Could you check a few things on this model? Use its own coordinates, in mm. A direction names the side the tool comes from. Give positions to 0.01 mm unless a question says otherwise; leave off trailing zeros. Loops run counter-clockwise (first coordinate to the right, second up) from the corner with the lowest first, then second, coordinate; pieces in that order, holes last. Notation, with made-up numbers: M 6,54.25 L 38,54.25 A23 ccw 38,93.25 Z; hole C -32,79.5 d8. An arc over 180 degrees is marked long. Use CSV: the item, a comma, the result in double quotes.
```python
from build123d import *

# Parameters (mm, degrees)
F1_DEPTH    = 30
F2_T1_DEPTH = 40
F3_T1_DEPTH = 40
F4_T1_DEPTH = 40


# Not quite as in the source:
# - a fillet or chamfer that OpenCascade refuses, or shapes differently, is made with other operations: its cross-section is extruded or revolved along the edge and cut away or added


with BuildPart() as f1:
    # F0 (on Top) → F1 (new body)
    with BuildSketch(Plane.XY):
        Polygon((-20, 3), (-23, 3), (-23, -12), (-20, -12), (-20, 0), (0, 0), (0, -12), (0, -24.0508113056), (3, -24.0508113056), (3, -12), (3, 0), (19, 0), (22, 0), (22, 22.2248057965), (19, 22.2248057965), (19, 3), (3, 3), (3, 22.2248057965), (0, 22.2248057965), (0, 3), align=None)
    extrude(amount=F1_DEPTH)

    # F2: fillet of radius 2 on 2 edges, made by hand

    # F2_s2 → F2_t1 (cut)
    with BuildSketch(Plane.XY.offset(-5)):
        with BuildLine():
            ThreePointArc((2, -24.0508113056), (0.5857864376, -23.465024868), (0, -22.0508113056))
            Line((0, -22.0508113056), (0, -24.0508113056))
            Line((0, -24.0508113056), (2, -24.0508113056))
        make_face()
        with BuildLine():
            ThreePointArc((3, -22.0508113056), (2.4142135624, -23.465024868), (1, -24.0508113056))
            Line((1, -24.0508113056), (3, -24.0508113056))
            Line((3, -24.0508113056), (3, -22.0508113056))
        make_face()
    extrude(amount=F2_T1_DEPTH, mode=Mode.SUBTRACT)

    # F3: fillet of radius 2 on 2 edges, made by hand

    # F3_s2 → F3_t1 (cut)
    with BuildSketch(Plane.XY.offset(-5)):
        with BuildLine():
            ThreePointArc((-23, -10), (-22.4142135624, -11.4142135624), (-21, -12))
            Line((-21, -12), (-23, -12))
            Line((-23, -12), (-23, -10))
        make_face()
        with BuildLine():
            ThreePointArc((-22, -12), (-20.5857864376, -11.4142135624), (-20, -10))
            Line((-20, -10), (-20, -12))
            Line((-20, -12), (-22, -12))
        make_face()
    extrude(amount=F3_T1_DEPTH, mode=Mode.SUBTRACT)

    # F4: fillet of radius 2 on 5 edges, made by hand

    # F4_s2 → F4_t1 (cut)
    with BuildSketch(Plane.XY.offset(-5)):
        with BuildLine():
            ThreePointArc((-21, 3), (-22.4142135624, 2.4142135624), (-23, 1))
            Line((-23, 1), (-23, 3))
            Line((-23, 3), (-21, 3))
        make_face()
        with BuildLine():
            ThreePointArc((0, 20.2248057965), (0.5857864376, 21.6390193588), (2, 22.2248057965))
            Line((2, 22.2248057965), (0, 22.2248057965))
            Line((0, 22.2248057965), (0, 20.2248057965))
        make_face()
        with BuildLine():
            ThreePointArc((19, 20.2248057965), (19.5857864376, 21.6390193588), (21, 22.2248057965))
            Line((21, 22.2248057965), (19, 22.2248057965))
            Line((19, 22.2248057965), (19, 20.2248057965))
        make_face()
        with BuildLine():
            ThreePointArc((1, 22.2248057965), (2.4142135624, 21.6390193588), (3, 20.2248057965))
            Line((3, 20.2248057965), (3, 22.2248057965))
            Line((3, 22.2248057965), (1, 22.2248057965))
        make_face()
        with BuildLine():
            ThreePointArc((20, 22.2248057965), (21.4142135624, 21.6390193588), (22, 20.2248057965))
            Line((22, 20.2248057965), (22, 22.2248057965))
            Line((22, 22.2248057965), (20, 22.2248057965))
        make_face()
    extrude(amount=F4_T1_DEPTH, mode=Mode.SUBTRACT)


solid = f1.part
```
1. I'm going to push flat-ended pins straight in: pin 1 Ø11 at (y, z) = (-10.5, 20) entering from +X; pin 2 Ø3 at (y, z) = (-13, 8) entering from -X; pin 3 Ø17 at (x, z) = (-10, 8.5) entering from +Y. Where does each tip first touch, or does it pass through?
Outcome:
pin 1,"x = 3"
pin 2,"x = -22.32"
pin 3,"y = 3"
2. I want a section at A-A, the plane y = -2.5. List the corners of the cut face in (x, z) for me, then the cut area to 3 significant figures.
Outcome:
outline,"M -23,0 L -20,0 L -20,30 L -23,30 Z; M 0,0 L 3,0 L 3,30 L 0,30 Z"
area,"180 mm2"
3. If we mould it in two halves opening along X, with no side actions, what happens to faces 1 (the face through (3, -11, 15)), 2 (the face through (11, 3, 15)), 3 (the face through (-10, 0, 15)), 4 (the face through (0, 12, 15))? For each: +X half, -X half, draft (parallel to the pull), parting line (faces both ways), or undercut.
Outcome:
face 1,"+X half"
face 2,"undercut"
face 3,"undercut"
face 4,"-X half"
4. I want a section at B-B, the plane z = 20. List the corners of the cut face in (x, y) for me, then the cut area to 3 significant figures.
Outcome:
outline,"M -23,-10 A2 ccw -21.5,-11.94 A2 ccw -20,-10 L -20,0 L 0,0 L 0,-22.05 A2 ccw 1.5,-23.99 A2 ccw 3,-22.05 L 3,0 L 22,0 L 22,20.22 A2 ccw 20.5,22.16 A2 ccw 19,20.22 L 19,3 L 3,3 L 3,20.22 A2 ccw 1.5,22.16 A2 ccw 0,20.22 L 0,3 L -21,3 A2 ccw -23,1 Z"
area,"351 mm2"
5. Please list where these lines run through material, in increasing order: line 1 (X direction, y = 17.5, z = 10.5); line 2 (Y direction, x = -5, z = 14.25); line 3 (X direction, y = -1, z = 26.5).
Outcome:
line 1,"0 to 3, 19 to 22"
line 2,"0 to 3"
line 3,"-23 to -20, 0 to 3"
6. Which directions (+Z, -Z, +X, -X, +Y, -Y) give clear straight access to the entire face, cutting with the end or side of a thin tool? Please do faces 5 (the face through (12, 0, 15)), 6 (the face through (-20.4, -11.2, 14.8)), 7 (the face through (19, 12, 15)), 8 (the face through (-10, 3, 15)).
Outcome:
face 5,"+Z, -Z, +X, -Y"
face 6,"+Z, -Z, -Y"
face 7,"+Z, -Z, +Y"
face 8,"+Z, -Z, -X, +Y"
7. I want a section at C-C, the plane x = 8. List the corners of the cut face in (y, z) for me.
Outcome:
outline,"M 0,0 L 3,0 L 3,30 L 0,30 Z"
